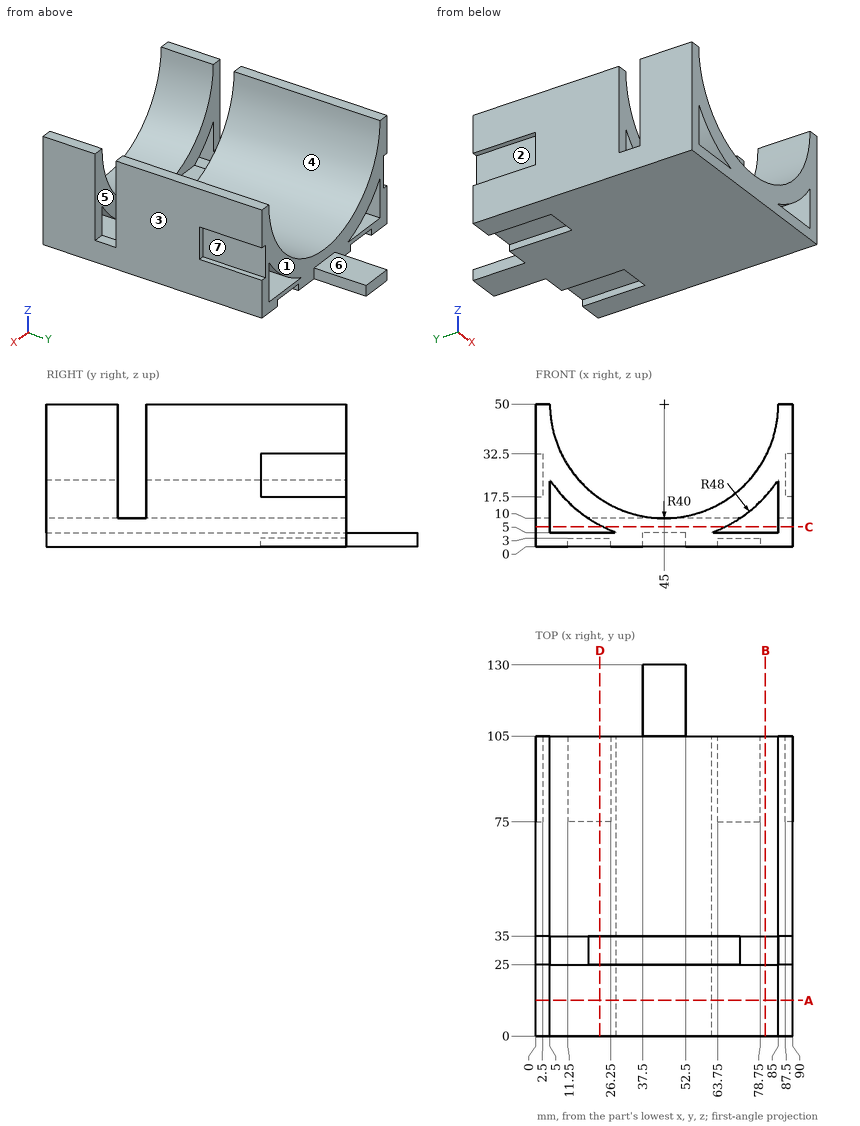
Geometry: see drawing. Coordinates: mm, zero at the bounding-box minimum. A direction names the side the tool comes from. Round coordinates to 2 decimals unless told otherwise and drop trailing zeros. Write each loop counter-clockwise with the first axis right and the second up, starting at its lowest first coordinate (ties: lowest second). Pieces come first, ordered by that corner, then holes.
1) Cut plane A-A (y = 12.5). Return the cut outline in (x, z), then the cut area to 3 significant figures.
2) Cut plane D-D (x = 22.5). Return the cut outline in (y, z), then the cut area to 3 significant figures.
3) Contact query for flat-ended pins moving along their axis: P1, Ø8, axis at x = 41.5, y = 28.5, coming from the +Z side; P2, Ø1.2, axis at x = 1, z = 27.5, coming from the +Y side; P3, Ø3, axis at x = 43.5, y = 62, coming from the +Z side. Output: stop coordinate, or through.
4) Cut plane C-C (z = 7). Return the cut outline in (x, y), then the cut area to 3 significant figures.
5) Cut plane B-B (x = 80.5). Return the cut outline in (y, z), then the cut area to 3 significant figures.
6) Draft query along X for the marked faces 1, 2, 3 and 4. Return one class per face: pulls with the +X half, pulls with the -X half, needs draft (parallel to the pull), parting line crosses it, or undercut.
7) Ray query, L1, parallel to X at y = 9, z = 15; L2, parallel to Y at x = 86, z = 18; L3, parallel to Z at x = 60, y = 32. Return the intervals inside material, ascending.
8) Reachability of the marked faces 5, 6 and 7 from +Z, -Z, +X, -X, +Y, -Y: full face, straight path, thin tool, end or side. Return the list, or none.
Geometry says:
1. outline: (0, 0) - (90, 0) - (90, 50) - (85, 50) arc R40 cw to (5, 50) - (0, 50) - close; hole (5, 5) - (28.3, 5) arc R48 cw to (5, 23.47) - close; hole (61.7, 5) - (85, 5) - (85, 23.47) arc R48 cw to start
1. area: 1,650 mm2
2. outline: (0, 0) - (75, 0) - (75, 3) - (105, 3) - (105, 5) - (0, 5) - close; (0, 7.6) - (105, 7.6) - (105, 16.93) - (35, 16.93) - (35, 10) - (25, 10) - (25, 16.93) - (0, 16.93) - close
2. area: 1,350 mm2
3. P1: stops at z = 10.37
3. P2: stops at y = 75
3. P3: stops at z = 10.11
4. outline: (0, 0) - (5, 0) - (5, 105) - (0, 105) - close; (23.67, 0) - (66.33, 0) - (66.33, 105) - (23.67, 105) - close; (85, 0) - (90, 0) - (90, 105) - (85, 105) - close
4. area: 5,530 mm2
5. outline: (0, 0) - (105, 0) - (105, 5) - (0, 5) - close; (0, 17.69) - (25, 17.69) - (25, 31.57) - (0, 31.57) - close; (35, 17.69) - (105, 17.69) - (105, 31.57) - (35, 31.57) - close
5. area: 1,840 mm2
6. face 1: needs draft
6. face 2: pulls with the -X half
6. face 3: pulls with the +X half
6. face 4: undercut
7. L1: x = 0 to 5, 12.15 to 25.64, 64.36 to 77.85, 85 to 90
7. L2: y = 0 to 25, 35 to 105
7. L3: z = 0 to 10
8. face 5: +Z, +X, -X
8. face 6: +Z, +X, -X, +Y
8. face 7: +X, +Y
